Input: part model. Units: mm. Frame: model coordinates. Face numbers are marked on the shaded views. Coordinates: 2 decimals unless noted, no trailing zeros. Order: outer loops, then holes, each group sorted by start corner. A loop starts at its lowest first (then second) coordinate and runs counter-clockwise, first axis right, second up. Notation, with made-up numbers: M 6.25,66 L 65.25,66 A38 cw 65.25,104 Z; hole C 33,75 d6. An arc over 180 degrees is marked long. Answer in a Markdown table with one row per item.
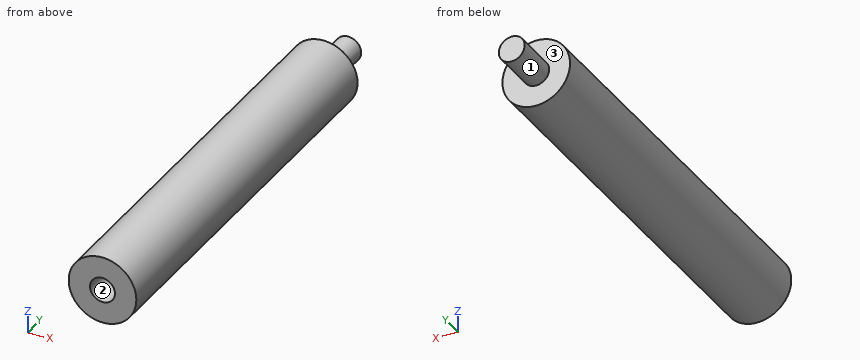
from build123d import *

# Parameters (mm, degrees)
SKETCH1_R           = 9.525
BOSS_EXTRUDE1_DEPTH = 114.3
SKETCH2_R           = 3.63855
BOSS_EXTRUDE2_DEPTH = 12.7
SKETCH3_R           = 3.51155
CUT_EXTRUDE1_DEPTH  = 12.7


with BuildPart() as part:
    # Sketch1 → Boss-Extrude1 (new body)
    with BuildSketch(Plane(origin=(0, 0, 0), x_dir=(1, 0, 0), z_dir=(0, 1, 0))):
        Circle(SKETCH1_R)
    extrude(amount=BOSS_EXTRUDE1_DEPTH)

    # Sketch2 → Boss-Extrude2 (add)
    with BuildSketch(Plane(origin=(0, 114.3, 0), x_dir=(1, 0, 0), z_dir=(0, 1, 0))):
        Circle(SKETCH2_R)
    extrude(amount=BOSS_EXTRUDE2_DEPTH)

    # Sketch3 → Cut-Extrude1 (cut)
    with BuildSketch(Plane.XZ):
        Circle(SKETCH3_R)
    extrude(amount=-CUT_EXTRUDE1_DEPTH, mode=Mode.SUBTRACT)


solid = part.part
1) Cut plane D-D, the plane x = 8. Output: boundary loops of the cut face in (y, z).
Resolved:
| item | result |
|---|---|
| outline | M 0,-5.17 L 114.3,-5.17 L 114.3,5.17 L 0,5.17 Z |
2) Mould query, pull axis Z, two halves, no side actions, for the marked faces 1, 2 and 3. Classes: +Z half, -Z half, draft (parallel to the pull), parting line (faces both ways), or undercut.
Resolved:
| item | result |
|---|---|
| face 1 | parting line |
| face 2 | undercut |
| face 3 | draft |
3) Cut plane A-A, the plane x = 0. Output: boundary loops of the cut face in (y, z) (3 decimals).
Resolved:
| item | result |
|---|---|
| outline | M 0,-9.525 L 114.3,-9.525 L 114.3,-3.639 L 127,-3.639 L 127,3.639 L 114.3,3.639 L 114.3,9.525 L 0,9.525 L 0,3.512 L 12.7,3.512 L 12.7,-3.512 L 0,-3.512 Z |
4) Contact query for flat-ended pins moving along their axis: pin 1 (1.5 mm diameter, centred on y = 81, z = 6.5, fed in from -X); pin 2 (4 mm diameter, centred on x = -6.5, z = -1, fed in from -Y); pin 3 (2 mm diameter, centred on y = 91.5, z = 5, fed in from +X); pin 4 (6.5 mm diameter, centred on x = 0, z = 0, fed in from -Y). Output: stop coordinate, or through.
Resolved:
| item | result |
|---|---|
| pin 1 | stops at x = -7.59 |
| pin 2 | stops at y = 0 |
| pin 3 | stops at x = 8.64 |
| pin 4 | stops at y = 12.7 |
5) Cut plane B-B, the plane z = 0. Output: boundary loops of the cut face in (x, y) (3 decimals).
Resolved:
| item | result |
|---|---|
| outline | M -9.525,0 L -3.512,0 L -3.512,12.7 L 3.512,12.7 L 3.512,0 L 9.525,0 L 9.525,114.3 L 3.639,114.3 L 3.639,127 L -3.639,127 L -3.639,114.3 L -9.525,114.3 Z |
6) Material intervals for probe 1 along Z at (x, y) = (0, 10.25) (3 decimals); probe 2 along Y at (x, z) = (5.75, 0.5); probe 3 along Y at (x, z) = (-1.25, 0.75), sorted ascending.
Resolved:
| item | result |
|---|---|
| probe 1 | z = -9.525 to -3.512, 3.512 to 9.525 |
| probe 2 | y = 0 to 114.3 |
| probe 3 | y = 12.7 to 127 |
7) Cut plane C-C, the plane y = 99. Output: boundary loops of the cut face in (x, z) (3 decimals).
Resolved:
| item | result |
|---|---|
| outline | C 0,0 d19.05 |
